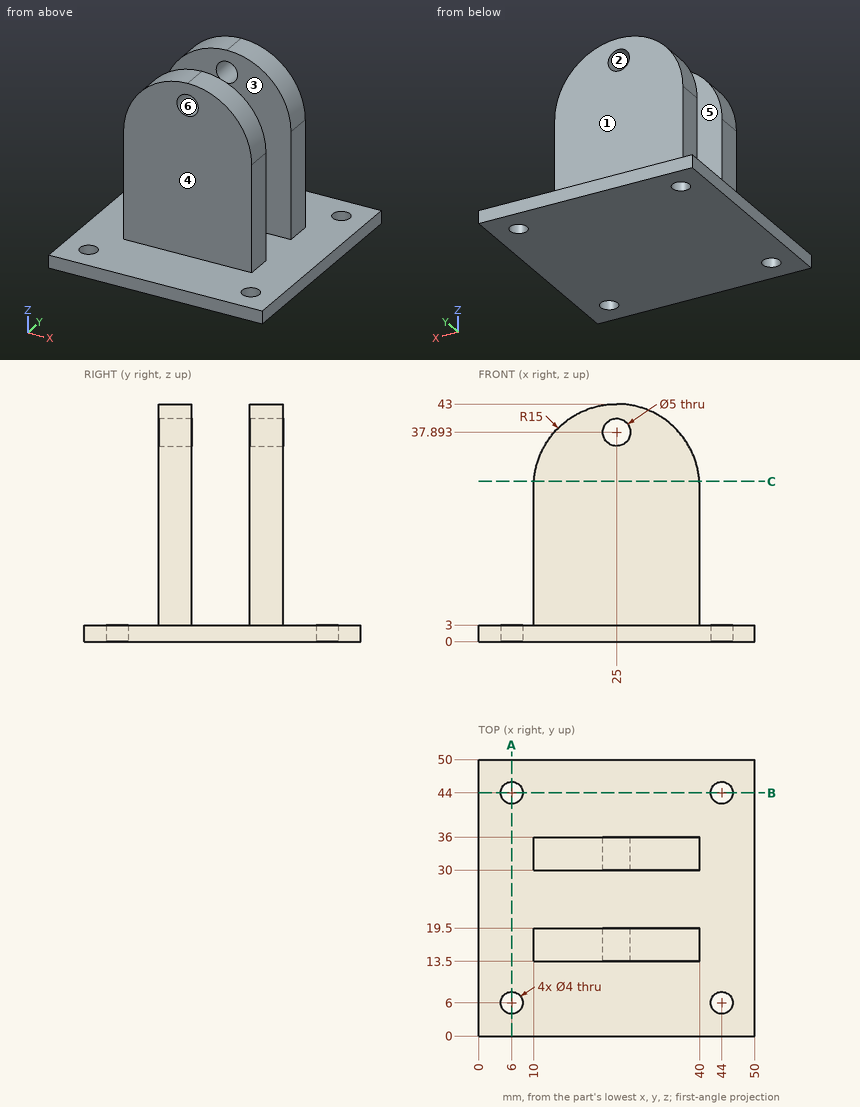
Design review of the part shown in the three views and the two pictorial views. Dimensions are in mm from the part's minimum x, y and z. A direction names the side the tool comes from. Coordinates: 2 decimals unless noted, no trailing zeros. Write each loop counter-clockwise with the first axis right and the second up, starting at its lowest first coordinate (ties: lowest second). Pieces come first, ordered by that corner, then holes. Notation, with made-up numbers: (-18.5, -10) -> (28.5, -10) arc R29 cw to (28.5, 27) -> close; hole circle Ø2 at (52.25, 68.5). An arc over 180 degrees is marked (long way). Answer in a Markdown table with one row per item.
1. We need section C-C, the plane z = 29. State the section outline as (x, y) points.
Answers below:
| item | result |
|---|---|
| outline | (10.03, 13.5) -> (39.97, 13.5) -> (39.97, 19.5) -> (10.03, 19.5) -> close; (10.03, 30) -> (39.97, 30) -> (39.97, 36) -> (10.03, 36) -> close |
2. Wall thickness on probe 1 along Y at (x, z) = (44, 1); probe 2 along Y at (x, z) = (27.5, 34.5); probe 3 along Z at (x, y) = (25, 15): over which ranges is each line inside the solid? List them lowest first. Write a range as [from, to].
Answers below:
| item | result |
|---|---|
| probe 1 | y = [0, 4], [8, 42], [46, 50] |
| probe 2 | y = [13.5, 19.5], [30, 36] |
| probe 3 | z = [0, 35.39], [40.39, 43] |
3. We need section A-A, the plane x = 6. State the section outline as (y, z) points.
Answers below:
| item | result |
|---|---|
| outline | (0, 0) -> (4, 0) -> (4, 3) -> (0, 3) -> close; (8, 0) -> (42, 0) -> (42, 3) -> (8, 3) -> close; (46, 0) -> (50, 0) -> (50, 3) -> (46, 3) -> close |
4. Clearance check with flat-ended pins moving along their axes: pin 1 Ø6.5 at (y, z) = (32, 12) entering from -X; pin 2 Ø1.8 at (y, z) = (16, 15) entering from +X; pin 3 Ø4.5 at (x, y) = (44, 44) entering from +Z; pin 4 Ø3 at (x, y) = (6, 44) entering from +Z. State where each tip first meets the part, or that it passes through.
Answers below:
| item | result |
|---|---|
| pin 1 | stops at x = 10 |
| pin 2 | stops at x = 40 |
| pin 3 | stops at z = 3 |
| pin 4 | passes through |
5. For the marked faces 4, 5 and 6, list the 3-axis set-ups (+Z, -Z, +X, -X, +Y, -Y) from which the entire face can be reached by the end or side of a thin tool; tool diameter is ignored.
Answers below:
| item | result |
|---|---|
| face 4 | +Z, +X, -X, -Y |
| face 5 | +Z, +X, -X |
| face 6 | +Y, -Y |
6. Draft analysis for pull direction Y (two halves, no side actions). For the marked faces 1, 2 and 3, state which applies: +Y half, -Y half, draft (parallel to the pull), parting line (faces both ways), or undercut.
Answers below:
| item | result |
|---|---|
| face 1 | +Y half |
| face 2 | draft |
| face 3 | undercut |
